Could you check a few things on this model? Use its own coordinates, in mm. A direction names the side the tool comes from. Give positions to 0.01 mm unless a question says otherwise; leave off trailing zeros. Loops run counter-clockwise (first coordinate to the right, second up) from the corner with the lowest first, then second, coordinate; pieces in that order, holes last.
1. Imagine slicing it at A-A (x = -16). List the corners of the cut face in (y, z) for me.
2. For P1, Ø1.5, axis at x = 24.5, z = 1.5, coming from the -Y side; P2, Ø1.5, axis at x = 27.5, z = 3.5, coming from the +Y side, each with a flat end and sliding along its axis, tell me the tip position at first contact or that it passes through.
3. I need wall thicknesses on line 1 along Y through (x, z) = (34, 3.7); line 2 along Y through (x, z) = (-14.5, 4); line 3 along Y through (x, z) = (-10.5, 2.45). Which ranges of each line are inside material? Lowest first, please.
4. For faces 1 (the cylindrical face through (-0.26, 19.483, 2.535)), 2 (the flat face through (30, 82, 3)), 3 (the flat face through (30, -123, 3)), which set-ups out of +Z, -Z, +X, -X, +Y, -Y let a thin tool reach every point of the face, with its end or its side?
5. Imagine slicing it at C-C (z = 3.1). Count the separate pieces of the cut face and the enclosed holes in it, plus the area to 3 significant figures.
6. Imagine slicing it at B-B (y = -52). List the corners of the cut face in (x, z) for me.
7. Imagine slicing it at D-D (x = 22.5). List the corners of the cut face in (y, z) for me.
8. Thinking about a two-plate mould opening in Y: for faces 4 (the flat face through (-10, -123, 3)), 5 (the cylindrical face through (34.923, -29.774, 2.535)), 6 (the flat face through (-20, 80, 3)), which applies, +Y half, -Y half, draft (parallel to the pull), parting line (faces both ways), or undercut?
```python
from build123d import *

# Parameters (mm, degrees)
SKETCH1_W           = 100
SKETCH1_H           = 210
BOSS_EXTRUDE1_DEPTH = 5
SKETCH4_W           = 20
SKETCH4_H           = 5
CUT_EXTRUDE3_DEPTH  = 10
SKETCH5_R           = 2
CUT_EXTRUDE4_DEPTH  = 6
SKETCH7_R           = 2
CUT_EXTRUDE5_DEPTH  = 10


with BuildPart() as part:
    # Sketch1 → Boss-Extrude1 (new body)
    with BuildSketch(Plane.XY):
        with Locations((0, -20)):
            Rectangle(SKETCH1_W, SKETCH1_H)
    extrude(amount=BOSS_EXTRUDE1_DEPTH)

    # Sketch4 → Cut-Extrude3 (cut)
    with BuildSketch(Plane.XY.offset(5)):
        with Locations((-20, 82.5)):
            Rectangle(SKETCH4_W, SKETCH4_H)
        with Locations((20, 82.5)):
            Rectangle(SKETCH4_W, SKETCH4_H)
        with Locations((20, -122.5)):
            Rectangle(SKETCH4_W, SKETCH4_H)
        with Locations((-20, -122.5)):
            Rectangle(SKETCH4_W, SKETCH4_H)
    extrude(amount=-CUT_EXTRUDE3_DEPTH, mode=Mode.SUBTRACT)

    # Sketch5 → Cut-Extrude4 (cut, through all)
    with BuildSketch(Plane.XY.offset(5)):
        with Locations((34, 52)):
            Circle(SKETCH5_R)
        with Locations((16, 52)):
            Circle(SKETCH5_R)
        with Locations((16, 28)):
            Circle(SKETCH5_R)
        with Locations((34, 28)):
            Circle(SKETCH5_R)
        with Locations((-16, 28)):
            Circle(SKETCH5_R)
        with Locations((-34, 28)):
            Circle(SKETCH5_R)
        with Locations((-34, 52)):
            Circle(SKETCH5_R)
        with Locations((-16, 52)):
            Circle(SKETCH5_R)
        with Locations((-16, -52)):
            Circle(SKETCH5_R)
        with Locations((-34, -52)):
            Circle(SKETCH5_R)
        with Locations((-34, -28)):
            Circle(SKETCH5_R)
        with Locations((-16, -28)):
            Circle(SKETCH5_R)
        with Locations((16, -28)):
            Circle(SKETCH5_R)
        with Locations((34, -28)):
            Circle(SKETCH5_R)
        with Locations((34, -52)):
            Circle(SKETCH5_R)
        with Locations((16, -52)):
            Circle(SKETCH5_R)
    extrude(amount=-CUT_EXTRUDE4_DEPTH, mode=Mode.SUBTRACT)

    # Sketch7 → Cut-Extrude5 (cut)
    with BuildSketch(Plane.XY.offset(5)):
        with Locations((0, 17.5)):
            Circle(SKETCH7_R)
        with Locations((0, -17.5)):
            Circle(SKETCH7_R)
    extrude(amount=-CUT_EXTRUDE5_DEPTH, mode=Mode.SUBTRACT)


solid = part.part
```
Derived:
1. outline: (-120, 0) - (-54, 0) - (-54, 5) - (-120, 5) - close; (-50, 0) - (-30, 0) - (-30, 5) - (-50, 5) - close; (-26, 0) - (26, 0) - (26, 5) - (-26, 5) - close; (30, 0) - (50, 0) - (50, 5) - (30, 5) - close; (54, 0) - (80, 0) - (80, 5) - (54, 5) - close
2. P1: stops at y = -120
2. P2: stops at y = 80
3. line 1: y = -125 to -54, -50 to -30, -26 to 26, 30 to 50, 54 to 85
3. line 2: y = -120 to -53.32, -50.68 to -29.32, -26.68 to 26.68, 29.32 to 50.68, 53.32 to 80
3. line 3: y = -120 to 80
4. face 1: +Z, -Z
4. face 2: +Z, -Z, +Y
4. face 3: +Z, -Z, -Y
5. separate pieces: 1
5. enclosed holes: 18
5. area: 20,400 mm2
6. outline: (-50, 0) - (-36, 0) - (-36, 5) - (-50, 5) - close; (-32, 0) - (-18, 0) - (-18, 5) - (-32, 5) - close; (-14, 0) - (14, 0) - (14, 5) - (-14, 5) - close; (18, 0) - (32, 0) - (32, 5) - (18, 5) - close; (36, 0) - (50, 0) - (50, 5) - (36, 5) - close
7. outline: (-120, 0) - (80, 0) - (80, 5) - (-120, 5) - close
8. face 4: draft
8. face 5: undercut
8. face 6: +Y half
